Build history of the part. All positions in model axes, mm. Coordinates: 2 decimals unless noted, no trailing zeros. Loops run counter-clockwise (first coordinate to the right, second up) from the corner with the lowest first, then second, coordinate; pieces in that order, holes last.
(1) Slice it at A-A (x = -40.5). Give the cut face in (y, z).
(2) Slice it at B-B (z = 2.7). Give the cut face in (x, y), and give its area (3 significant figures).
(3) Flat gauge pins, fed straight in: P1, Ø1, axis at x = -47, z = 4, coming from the -Y side; P2, Ø2.5, axis at y = -4, z = 3.5, coming from the +X side; P3, Ø2.5, axis at x = -11.5, z = 2, coming from the +Y side. Where does each tip first touch, or does it go through?
(4) Slice it at C-C (y = 3.5). Give the cut face in (x, z).
(5) Wall check: L1, parallel to Y at x = -23, z = 2.5; L2, parallel to X at y = -5, z = 2.15; L3, parallel to Y at x = 49.5, z = 2.3. Give the ranges that are in metal, low to high.
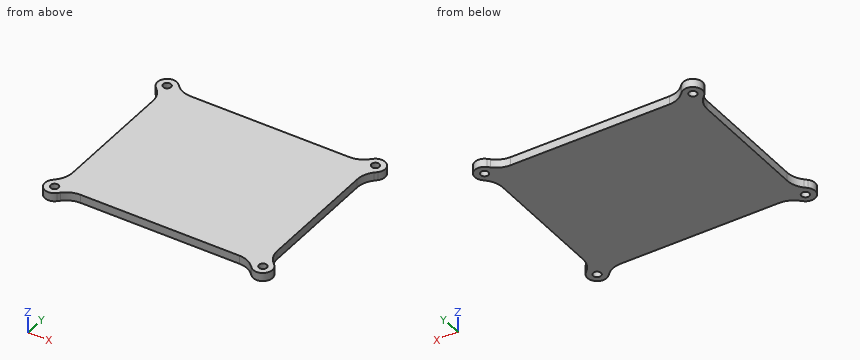
from build123d import *

# Parameters (mm, degrees)
BOSS_EXTRUDE1_DEPTH  = 4.7625
M4_CLEARANCE_HOLE1_D = 4.5


with BuildPart() as part:
    # Sketch2 → Boss-Extrude1 (new body)
    with BuildSketch(Plane.XY):
        with BuildLine():
            Line((-63.385065828, 38.234139131), (-62.103242019, 36.952315321))
            ThreePointArc((-62.103242019, 36.952315321), (-59.350228077, 32.832138791), (-58.38349814, 27.9720592))
            Line((-58.38349814, 27.9720592), (-58.38349814, -41.67556713))
            ThreePointArc((-58.38349814, -41.67556713), (-59.350228077, -46.535646721), (-62.103242019, -50.655823251))
            Line((-62.103242019, -50.655823251), (-63.385065828, -51.93764706))
            ThreePointArc((-63.385065828, -51.93764706), (-63.385065828, -59.715821653), (-55.606891235, -59.715821653))
            Line((-55.606891235, -59.715821653), (-54.325067426, -58.433997844))
            ThreePointArc((-54.325067426, -58.433997844), (-50.204890896, -55.680983902), (-45.344811305, -54.714253965))
            Line((-45.344811305, -54.714253965), (44.940315025, -54.714253965))
            ThreePointArc((44.940315025, -54.714253965), (49.800394616, -55.680983902), (53.920571146, -58.433997844))
            Line((53.920571146, -58.433997844), (55.202394956, -59.715821653))
            ThreePointArc((55.202394956, -59.715821653), (62.980569549, -59.715821653), (62.980569549, -51.93764706))
            Line((62.980569549, -51.93764706), (61.698745739, -50.655823251))
            ThreePointArc((61.698745739, -50.655823251), (58.945731797, -46.535646721), (57.97900186, -41.67556713))
            Line((57.97900186, -41.67556713), (57.97900186, 27.9720592))
            ThreePointArc((57.97900186, 27.9720592), (58.945731797, 32.832138791), (61.698745739, 36.952315321))
            Line((61.698745739, 36.952315321), (62.980569549, 38.234139131))
            ThreePointArc((62.980569549, 38.234139131), (62.980569549, 46.012313724), (55.202394956, 46.012313724))
            Line((55.202394956, 46.012313724), (53.920571146, 44.730489914))
            ThreePointArc((53.920571146, 44.730489914), (49.800394616, 41.977475972), (44.940315025, 41.010746035))
            Line((44.940315025, 41.010746035), (-45.344811305, 41.010746035))
            ThreePointArc((-45.344811305, 41.010746035), (-50.204890896, 41.977475972), (-54.325067426, 44.730489914))
            Line((-54.325067426, 44.730489914), (-55.606891235, 46.012313724))
            ThreePointArc((-55.606891235, 46.012313724), (-63.385065828, 46.012313724), (-63.385065828, 38.234139131))
        make_face()
    extrude(amount=BOSS_EXTRUDE1_DEPTH)

    # M4 Clearance Hole1 (through all)
    with Locations(Plane.XY.offset(4.7625)):
        with Locations((-59.495978532, -55.826734357), (-59.495978532, 42.123226427), (59.091482252, 42.123226427), (59.091482252, -55.826734357)):
            Hole(M4_CLEARANCE_HOLE1_D / 2)


solid = part.part
Response values:
1. outline: (-54.71, 0) - (41.01, 0) - (41.01, 4.76) - (-54.71, 4.76) - close
2. outline: (-63.39, -51.94) arc R5.5 ccw to (-55.61, -59.72) - (-54.33, -58.43) arc R12.7 cw to (-45.34, -54.71) - (44.94, -54.71) arc R12.7 cw to (53.92, -58.43) - (55.2, -59.72) arc R5.5 ccw to (62.98, -51.94) - (61.7, -50.66) arc R12.7 cw to (57.98, -41.68) - (57.98, 27.97) arc R12.7 cw to (61.7, 36.95) - (62.98, 38.23) arc R5.5 ccw to (55.2, 46.01) - (53.92, 44.73) arc R12.7 cw to (44.94, 41.01) - (-45.34, 41.01) arc R12.7 cw to (-54.33, 44.73) - (-55.61, 46.01) arc R5.5 ccw to (-63.39, 38.23) - (-62.1, 36.95) arc R12.7 cw to (-58.38, 27.97) - (-58.38, -41.68) arc R12.7 cw to (-62.1, -50.66) - close; hole circle Ø4.5 at (-59.5, -55.83); hole circle Ø4.5 at (-59.5, 42.12); hole circle Ø4.5 at (59.09, -55.83); hole circle Ø4.5 at (59.09, 42.12)
2. area: 11,500 mm2
3. P1: stops at y = -54.9
3. P2: stops at x = 57.98
3. P3: stops at y = 41.01
4. outline: (-58.38, 0) - (57.98, 0) - (57.98, 4.76) - (-58.38, 4.76) - close
5. L1: y = -54.71 to 41.01
5. L2: x = -58.38 to 57.98
5. L3: y = -55.56 to 41.86
